Can you work these out from the model? Positions are in its coordinate system, mm. A direction names the side the tool comes from. Round coordinates to 2 decimals unless told otherwise and drop trailing zeros. Write each loop counter-clockwise with the first axis right and the second up, starting at its lowest first coordinate (ties: lowest second). Pieces come first, ordered by that corner, then holes. Notation, with made-up numbers: M 85.25,-8.5 L 131.25,-8.5 A27 cw 131.25,22.5 Z; hole C 66,36.5 d3. An arc over 180 degrees is marked long. Answer as a JSON object with one key per item and string values. Group by question number.
1) On a 3-axis mill with a long thin cutter (end or side, diameter ignored), from which of +Z, -Z, +X, -X, +Y, -Y can I reach the whole of each face in a straight line? I mean faces 5 (the flat face through (-7, -4, 21)), 6 (the cylindrical face through (4.743, 0.488, 18.304)), 7 (the flat face through (2, -7, 15)), 8 (the flat face through (-2.155, -3.663, 12.415)), 9 (the flat face through (4, -4, 25)). Say none if no direction works.
2) Suppose I cut it at D-D, the plane z = 16.5. Write out the boundary of the cut face in (x, y).
3) I'm going to push flat-ended pins straight in: pin 1 Ø2 at (x, z) = (6.5, 21) entering from -Y; pin 2 Ø3 at (x, z) = (-1.5, 11.5) entering from +Y; pin 3 Ø5 at (x, z) = (7, 15) entering from +Y. Where does each tip first touch, or does it pass through?
4) If we mould it in two halves opening along X, with no side actions, what happens to faces 1 (the flat face through (6, 0, 17)), 2 (the flat face through (3, -4, 0)), 3 (the flat face through (-2.095, 3.698, 12.415)), 4 (the cylindrical face through (5.05, 4.63, 7.65))? For each: +X half, -X half, draft (parallel to the pull), parting line (faces both ways), or undercut.
5) Suppose I cut it at A-A, the plane z = 3. Write out the boundary of the cut face in (x, y).
6) Suppose I cut it at C-C, the plane y = 0. State how many separate pieces and enclosed holes the cut face has, and give its area (3 significant figures).
7) Please list where these lines run through material, in increasing order: L1, parallel to X at y = 2.25, z = 15.25; L2, parallel to X at y = -1.5, z = 4.75; L3, parallel to Z at x = 3.25, y = 7.25. Write a range as [from, to].
from build123d import *

# Parameters (mm, degrees)
F3_DEPTH = 25.001
F2_W     = 2.5
F2_H     = 8
F4_DEPTH = 8
F5_R     = 2.25
F6_DEPTH = 25
F7_SIZE  = 0.99999
F8_SIZE  = 0.5


# Not quite as in the source:
# - a fillet or chamfer is up to 0.001 mm smaller than in the source, because OpenCascade refuses the exact size


with BuildPart() as f1:
    # F0 (on Front) → F1 (revolve)
    with BuildSketch(Plane.XZ):
        Polygon((-6.85, 0), (0, 0), (0, 25), (-10, 25), (-10, 15), (-6.85, 15), align=None)
    revolve(axis=Axis((0, 0, 12.5), (0, 0, -1)))

    # F2 (on face) → F3 (cut, through all)
    with BuildSketch(Plane.XY.offset(25)):
        Polygon((4.25, -2.4537386441), (4.25, 2.4537386441), (0, 4.9074772881), (-4.25, 2.4537386441), (-4.25, -2.4537386441), (0, -4.9074772881), align=None)
    extrude(amount=-F3_DEPTH, mode=Mode.SUBTRACT)

    # F2 (on face) → F4 (cut)
    with BuildSketch(Plane.XY.offset(25)):
        with Locations((-6.5, 0)):
            Rectangle(F2_W, F2_H)
        with Locations((6.5, 0)):
            Rectangle(F2_W, F2_H)
    extrude(amount=-F4_DEPTH, mode=Mode.SUBTRACT)

    # F5 (on face) → F6 (cut, symmetric)
    with BuildSketch(Plane(origin=(-5.25, 0, 0), x_dir=(0, -1, 0), z_dir=(-1, 0, 0))):
        with Locations((0, 20.5)):
            Circle(F5_R)
    extrude(amount=F6_DEPTH, both=True, mode=Mode.SUBTRACT)

    # F7 (size 1 in the source; OpenCascade refuses exactly that, so slightly less here)
    f7_edges = [f1.edges().sort_by_distance(p)[0] for p in [
        (10, 0, 25),
        (10, 0, 15),
        (-2.125, 3.680608, 25),
        (2.125, 3.680608, 25),
        (4.25, 0, 25),
        (2.125, -3.680608, 25),
        (-2.125, -3.680608, 25),
        (-4.25, 0, 25),
    ]]
    chamfer(f7_edges, length=F7_SIZE)

    # F8
    f8_edges = [f1.edges().sort_by_distance(p)[0] for p in [
        (6.85, 0, 0),
        (4.25, 0, 0),
        (2.125, -3.680608, 0),
        (-2.125, -3.680608, 0),
        (-4.25, 0, 0),
        (-2.125, 3.680608, 0),
        (2.125, 3.680608, 0),
    ]]
    chamfer(f8_edges, length=F8_SIZE)


solid = f1.part
Results:
{
 "1": {"face 5": "+Z", "face 6": "+X, -X", "face 7": "-Z", "face 8": "+Z, -Z", "face 9": "+Z, +X, -X, +Y, -Y"},
 "2": {"outline": "C 0,0 d20; hole M -4.25,-2.45 L 0,-4.91 L 4.25,-2.45 L 4.25,2.45 L 0,4.91 L -4.25,2.45 Z"},
 "3": {"pin 1": "y = -8.35", "pin 2": "y = 6.85", "pin 3": "y = 8.82"},
 "4": {"face 1": "undercut", "face 2": "draft", "face 3": "undercut", "face 4": "parting line"},
 "5": {"outline": "C 0,0 d13.7; hole M -4.25,-2.45 L 0,-4.91 L 4.25,-2.45 L 4.25,2.45 L 0,4.91 L -4.25,2.45 Z"},
 "6": {"separate pieces": "6", "enclosed holes": "0", "area": "120 mm^2"},
 "7": {"L1": "[-8.97, -4.25], [4.25, 8.97]", "L2": "[-6.68, -4.25], [4.25, 6.68]", "L3": "[15, 25]"}
}
